```python
from build123d import *

# Parameters (mm, degrees)
SKETCH007_R     = 13
PAD003_DEPTH    = 3
PAD004_DEPTH    = 57.5
PAD005_DEPTH    = 57.5
SKETCH010_R     = 3
POCKET002_DEPTH = 37.501
SKETCH011_R     = 3
POCKET003_DEPTH = 37.501


with BuildPart() as part:
    # Sketch007 → Pad003 (new body)
    with BuildSketch(Plane.XY.offset(3)):
        with BuildLine():
            ThreePointArc((-20, 0), (-14.142136, -14.142136), (0, -20))
            Line((37.5, -20), (0, -20))
            Line((37.5, 37.5), (37.5, -20))
            Line((0, 37.5), (37.5, 37.5))
            Line((0, 37.5), (-20, 37.5))
            Line((-20, 37.5), (-20, 0))
        make_face()
        Circle(SKETCH007_R, mode=Mode.SUBTRACT)
    extrude(amount=PAD003_DEPTH)

    # Sketch008 → Pad004 (join)
    with BuildSketch(Plane.XZ.offset(20)):
        with BuildLine():
            Line((32.5, 3), (37.5, 3))
            Line((37.5, 3), (37.5, -10))
            Line((37.5, -10), (33.5, -10))
            Line((33.5, -10), (33.5, 2))
            ThreePointArc((33.5, 2), (33.207107, 2.707107), (32.5, 3))
        make_face()
    extrude(amount=-PAD004_DEPTH)

    # Sketch009 → Pad005 (join)
    with BuildSketch(Plane.YZ.offset(-20)):
        with BuildLine():
            Line((32.5, 3), (37.5, 3))
            Line((37.5, 3), (37.5, -10))
            Line((37.5, -10), (33.5, -10))
            Line((33.5, -10), (33.5, 2))
            ThreePointArc((33.5, 2), (33.207107, 2.707107), (32.5, 3))
        make_face()
    extrude(amount=PAD005_DEPTH)

    # Sketch010 → Pocket002 (cut, through all)
    with BuildSketch(Plane.YZ):
        with Locations((0, -4.137609)):
            Circle(SKETCH010_R)
    extrude(amount=POCKET002_DEPTH, mode=Mode.SUBTRACT)

    # Sketch011 → Pocket003 (cut, through all)
    with BuildSketch(Plane.XZ):
        with Locations((0, -4.137609)):
            Circle(SKETCH011_R)
    extrude(amount=-POCKET003_DEPTH, mode=Mode.SUBTRACT)


with BuildPart() as part_1:
    # Body001 placement: moved
    add(part.part.moved(Location((4, 0, 0))))


solid = part_1.part
```
The listing builds one solid part. Answer for the finished solid, in the listing's coordinates (mm). A direction names the side the tool comes from. Coordinates: 2 decimals unless noted, no trailing zeros. Order: outer loops, then holes, each group sorted by start corner. A loop starts at its lowest first (then second) coordinate and runs counter-clockwise, first axis right, second up. Notation, with made-up numbers: M 12.25,74.5 L 70.25,74.5 A11 cw 70.25,84.5 Z; hole C 37.5,-37.5 d2. An arc over 180 degrees is marked long. Answer as a JSON object with one key per item and string values. Group by question number.
1. Section B-B on y = -9 is taken. Write down the section's boundary in (x, z), then the cut area to 3 significant figures.
2. Flat-ended cylindrical pins translate along their axes: P1, Ø9.5, axis at y = 15, z = -2.5, coming from the -X side; P2, Ø5, axis at x = -6, z = -1, coming from the -Y side; P3, Ø10, axis at x = 31, y = 13.5, coming from the -Z side. Find the tip coordinate at first contact, or state that the pin passes through.
3. Determine the mould class of faces 1 (the cylindrical face through (1.003, 35.472, -4.006)), 2 (the flat face through (25, 34, -10)), 3 (the flat face through (-16, 23, 3.4)) for opening direction X: released by +X, released by -X, zero draft, split by the parting line, or undercut.
4. A tool of negligible diameter and unlimited length cuts with its end or side. For faces 4 (the flat face through (37.5, 6, -4)), 5 (the flat face through (12, 37.5, -2)), from which of +Z, -Z, +X, -X, +Y, -Y can it reach the whole face along a straight path? Write none if from no direction.
5. Section A-A on x = 0 is taken. Write down the section's boundary in (y, z).
6. Straight lines are drawn through the part: line 1 (Z direction, x = 40.05, y = 0); line 2 (X direction, y = 23, z = -1); line 3 (Z direction, x = 16, y = 16). For each, find the intervals that lie inside material, in ascending order.
7. Section D-D on x = 23 is taken. Write down the section's boundary in (y, z), then the cut area to 3 significant figures.
8. Section C-C on z = -8 is taken. Write down the section's boundary in (x, y), then the cut area to 3 significant figures.
Values follow:
{
 "1": {"outline": "M -13.86,3 L -5.38,3 L -5.38,6 L -13.86,6 Z; M 13.38,3 L 36.5,3 A1 cw 37.5,2 L 37.5,-10 L 41.5,-10 L 41.5,6 L 13.38,6 Z", "area": "162 mm2"},
 "2": {"P1": "x = 37.47", "P2": "y = 33.5", "P3": "z = 3"},
 "3": {"face 1": "undercut", "face 2": "zero draft", "face 3": "released by -X"},
 "4": {"face 4": "-Z, -X, -Y", "face 5": "+Z, -Z, +X, -X, +Y"},
 "5": {"outline": "M -19.6,3 L -12.37,3 L -12.37,6 L -19.6,6 Z; M 12.37,3 L 32.5,3 A1 cw 33.5,2 L 33.5,-10 L 37.5,-10 L 37.5,6 L 12.37,6 Z"},
 "6": {"line 1": "-10 to -7.14, -1.14 to 6", "line 2": "37.5 to 41.5", "line 3": "3 to 6"},
 "7": {"outline": "M -20,3 L 32.5,3 A1 cw 33.5,2 L 33.5,-10 L 37.5,-10 L 37.5,6 L -20,6 Z", "area": "225 mm2"},
 "8": {"outline": "M -16,33.5 L 37.5,33.5 L 37.5,-20 L 41.5,-20 L 41.5,37.5 L -16,37.5 Z", "area": "444 mm2"}
}
